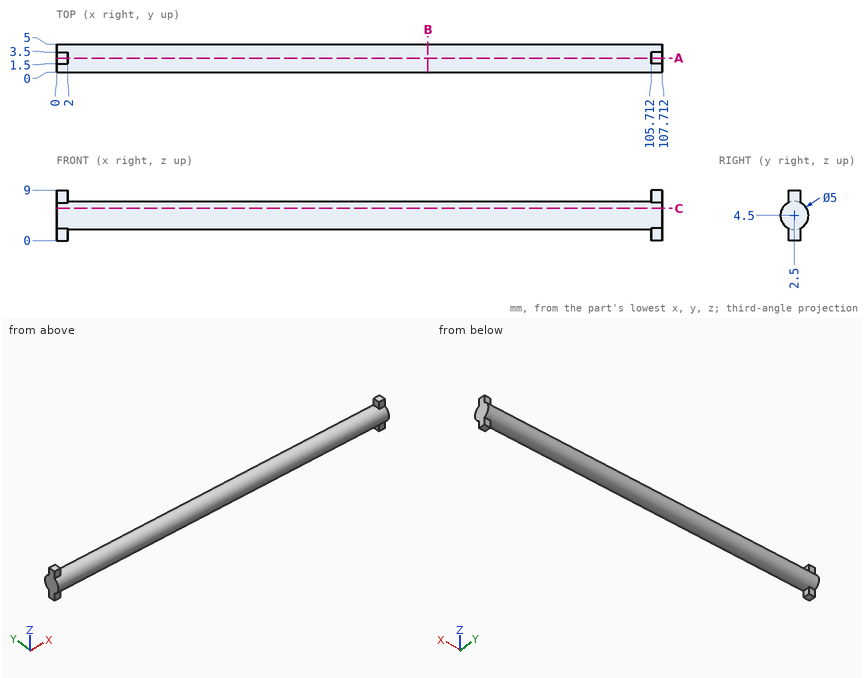
The drawing under review shows one solid part. Ordinate dimensions are in mm from its lowest x, y, z. Give positions to 0.01 mm unless a question says otherwise; leave off trailing zeros. Write each loop counter-clockwise with the first axis right and the second up, starting at its lowest first coordinate (ties: lowest second). Pieces come first, ordered by that corner, then holes. Notation, with made-up numbers: (44, 21) -> (56, 21) arc R22 cw to (56, 30) -> close; hole circle Ø1 at (-36.5, -32). An arc over 180 degrees is marked (long way). Answer in a Markdown table with one row per item.
(1) Clearance check with flat-ended pins moving along their axes: pin 1 (2 mm diameter, centred on x = 44.5, z = 7, fed in from -Y); pin 2 (1 mm diameter, centred on x = 1.5, z = 1, fed in from -Y); pin 3 (0.6 mm diameter, centred on x = 106.5, z = 0.5, fed in from +Y). State where each tip first meets the part, or that it passes through.
Results:
| item | result |
|---|---|
| pin 1 | y = 0.5 |
| pin 2 | y = 1.5 |
| pin 3 | y = 3.5 |
(2) Consider section B-B (x = 66). State the section outline as (y, z) points.
Results:
| item | result |
|---|---|
| outline | circle Ø5 at (2.5, 4.5) |
(3) To check wall thickness, follow probe 1 along Z at (x, y) = (70.5, 2.35); probe 2 along Y at (x, z) = (83.5, 4.25); probe 3 along Z at (x, y) = (89, 0.9). State the ranges of each line that lie inside material, in increasing order.
Results:
| item | result |
|---|---|
| probe 1 | 2 to 7 |
| probe 2 | 0.01 to 4.99 |
| probe 3 | 2.58 to 6.42 |
(4) Consider section C-C (z = 5.75). State the section outline as (x, y) points, then the cut area to 3 significant figures.
Results:
| item | result |
|---|---|
| outline | (0, 0.33) -> (107.71, 0.33) -> (107.71, 4.67) -> (0, 4.67) -> close |
| area | 466 mm2 |
(5) Consider section A-A (y = 2.5). State the section outline as (x, z) points, then the cut area to 3 significant figures.
Results:
| item | result |
|---|---|
| outline | (0, 0) -> (2, 0) -> (2, 2) -> (105.71, 2) -> (105.71, 0) -> (107.71, 0) -> (107.71, 9) -> (105.71, 9) -> (105.71, 7) -> (2, 7) -> (2, 9) -> (0, 9) -> close |
| area | 555 mm2 |
